Verification items for the finished model (mm, model axes). A direction names the side the tool comes from. Give positions to 0.01 mm unless a question says otherwise; leave off trailing zeros. Write each loop counter-clockwise with the first axis right and the second up, starting at its lowest first coordinate (ties: lowest second). Pieces come first, ordered by that corner, then holes. Notation, with made-up numbers: (52.5, 52.5) -> (81.5, 52.5) arc R26 cw to (81.5, 67.5) -> close; hole circle Ø11 at (2.25, -15.75). An arc over 180 degrees is marked (long way). Use one line per item in the form item = value. Start each with the question number.
(1) Depth check by flat-ended pin: pin 1 Ø3 at (x, y) = (-10.5, 1) entering from -Z; pin 2 Ø4 at (x, y) = (-5.5, 3.5) entering from -Z; pin 3 Ø2 at (x, y) = (-2, -1.5) entering from +Z. Enter the tip coordinate at first touch or a pass-through.
(2) Section check A-A, the plane x = -12.5. Record the cut outline in (y, z), plus the area to 3 significant figures.
(3) Scan lines: L1, parallel to Y at x = -2.5, z = 2.5; L2, parallel to Y at x = -11.5, z = -1.75; L3, parallel to X at y = 0.5, z = -1.25. Record each from-to range of solid material in increasing order.
(4) Set-up check for faces 1 (the face through (14, 0, 0)), 2 (the face through (-2, -3, 0)): record each of +Z, -Z, +X, -X, +Y, -Y from which the full face is reachable in a straight line by a thin tool's end or side.
Autodesk Fusion 360 part; units mm, degrees
sketch "Sketch1" plane through (0, 0, 0) normal (1, 0, 0) x (0, 1, 0)
  circle A0 centre (0, 0) radius 3
  dimension "d1" = 6
extrude "Extrude1" add sketch "Sketch1" against normal blind 15
extrude "Extrude2" add 1 faces at (0, -1.1591, 0.5829) along direction (1, 0, 0) blind 10
sketch "Sketch2" plane through (10, 0, 0) normal (1, 0, 0) x (0, 1, 0)
  circle A0 centre (0, 0) radius 3
  circle A1 centre (0, 0) radius 5
  dimension "d7" = 10
extrude "Extrude3" add sketch "Sketch2" along normal blind 4 contours A0 | A1
fillet "Fillet1" radius 4 1 edges at (14, -4.6616, -1.8081)
thread "Thread1"
Completed:
q1.pin_1 = -3
q1.pin_2 = -2.6
q1.pin_3 = 2.96
q2.outline = circle Ø6 at (0, 0)
q2.area = 28.3 mm²
q3.L1 = -1.66 to 1.66
q3.L2 = -2.44 to 2.44
q3.L3 = -15 to 13.99
q4.face_1 = +Z, -Z, +X, +Y, -Y
q4.face_2 = -X
